Source: CAD feature listing. Evaluate the final solid. Frame: model axes, mm. Face numbers are marked on the shaded views. Coordinates: 2 decimals unless noted, no trailing zeros. Write each loop counter-clockwise with the first axis right and the second up, starting at its lowest first coordinate (ties: lowest second). Pieces come first, ordered by that corner, then holes. Notation, with made-up numbers: (68.25, 26.5) - (94.25, 26.5) arc R33 cw to (94.25, 56.5) - close; hole circle Ø1 at (51.5, 77). An arc over 180 degrees is marked (long way). One line per item, written item: value.
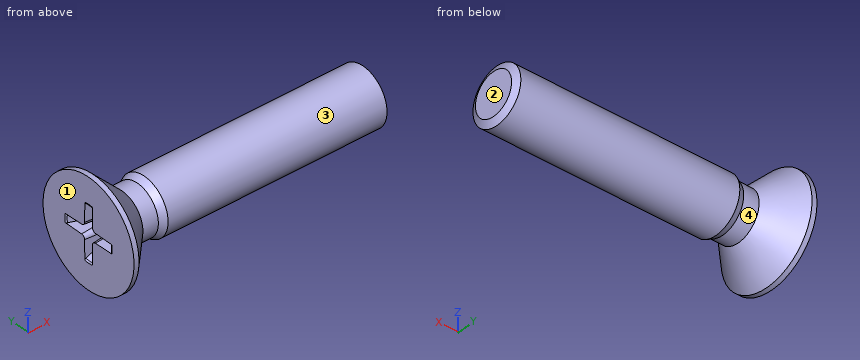
Autodesk Inventor part; units mm, degrees
ref_plane "Work Plane2" through (3.35, 0, 0) normal (0, 0, -1) x (1, 0, 0)
ref_plane "YZ Plane" through (0, 0, 0) normal (1, 0, 0) x (0, 1, 0)
ref_plane "XZ Plane" through (0, 0, 0) normal (0, 1, 0) x (-1, 0, 0)
sketch "Skizze1" plane through (0, 0, 0) normal (0, 0, 1) x (1, 0, 0)
  line L0 (1.2, 0) -> (10, 0)
  line L1 (10, 0) -> (10, 1)
  line L2 (10, 1) -> (2, 1)
  line L3 (2, 1) -> (1.7546, 0.8773)
  line L4 (1.7546, 0.8773) -> (1.2, 0.8773)
  line L5 (0, 1.9) -> (0, 0.95)
  line L6 (0, 0.95) -> (0.9455, 0.4786)
  line L7 (0.9455, 0.4786) -> (1.2, 0)
  line L8 (-2, 0) -> (12, 0)
  line L9 (0, -0.38) -> (0, 2.28)
  line L10 (0, 1.9) -> (0.1773, 1.9)
  line L11 (0.1773, 1.9) -> (1.2, 0.8773)
  line L12 (2, 1) -> (1.0773, 1) construction
  dimension "d1" = 8
  dimension "d2" = 2
  dimension "d3" = 1.7546
  dimension "d4" = 1.9
  dimension "d5" = 26.5
  dimension "d6" = 62
  dimension "d7" = 1.2
  dimension "d8" = 0.2454
  dimension "d12" = 3.8
  dimension "d13" = 45
  dimension "d15" = 10
  dimension "d24" = 1.2
revolve "Körper" add sketch "Skizze1" angle 360 about axis through (1.2, 0, 0) along (1, 0, 0) contours L7 L6 L5 L10 L11 L4 L3 L2 L1 L0
sketch "Skizze2" plane through (0, 0, 0) normal (-1, 0, 0) x (0, 0, 1)
  line L0 (0, 0.95) -> (0, 0) construction
  line L1 (0, 0) -> (0.95, 0) construction
  arc A0 (0.285, 0) -> (0, 0.285) centre (0, 0) ccw construction
  arc A1 (0.3325, 0) -> (0, 0.3325) centre (0, 0) ccw construction
  arc A2 (0.9373, 0.155) -> (0.155, 0.9373) centre (0, 0) ccw
  line L2 (0, 0) -> (0.6718, 0.6718) construction
  line L3 (0.155, 0.9373) -> (0.1646, 0.2889)
  line L4 (0.9373, 0.155) -> (0.2889, 0.1646)
  arc A3 (0.155, 0.9373) -> (0, 0.95) centre (0, 0) ccw
  arc A4 (0.95, 0) -> (0.9373, 0.155) centre (0, 0) ccw
  line L5 (0, -2.66) -> (0, 2.66)
  line L6 (-2.66, 0) -> (2.66, 0)
  arc A5 (0.155, -0.9373) -> (0.9373, -0.155) centre (0, 0) ccw
  line L7 (0.155, -0.9373) -> (0.1646, -0.2889)
  line L8 (0.9373, -0.155) -> (0.2889, -0.1646)
  arc A6 (0, -0.95) -> (0.155, -0.9373) centre (0, 0) ccw
  arc A7 (0.9373, -0.155) -> (0.95, 0) centre (0, 0) ccw
  arc A8 (-0.155, 0.9373) -> (-0.9373, 0.155) centre (0, 0) ccw
  line L9 (-0.155, 0.9373) -> (-0.1646, 0.2889)
  line L10 (-0.9373, 0.155) -> (-0.2889, 0.1646)
  arc A9 (0, 0.95) -> (-0.155, 0.9373) centre (0, 0) ccw
  arc A10 (-0.9373, 0.155) -> (-0.95, 0) centre (0, 0) ccw
  arc A11 (-0.155, -0.9373) -> (0, -0.95) centre (0, 0) ccw
  arc A12 (-0.9373, -0.155) -> (-0.155, -0.9373) centre (0, 0) ccw
  arc A13 (-0.95, 0) -> (-0.9373, -0.155) centre (0, 0) ccw
  line L11 (-0.9373, -0.155) -> (-0.2889, -0.1646)
  line L12 (-0.155, -0.9373) -> (-0.1646, -0.2889)
  arc A14 (0.1646, 0.2889) -> (0.2889, 0.1646) centre (0.2908, 0.2908) ccw
  arc A15 (0.2889, -0.1646) -> (0.1646, -0.2889) centre (0.2908, -0.2908) ccw
  arc A16 (-0.2889, 0.1646) -> (-0.1646, 0.2889) centre (-0.2908, 0.2908) ccw
  arc A17 (-0.1646, -0.2889) -> (-0.2889, -0.1646) centre (-0.2908, -0.2908) ccw
  point P0 (0.6718, -0.6718)
  point P1 (-0.6718, 0.6718)
  point P2 (-0.6718, -0.6718)
  dimension "d17" = 0.57
  dimension "d18" = 0.665
  dimension "d19" = 1.9
  dimension "d20" = 45
  dimension "d21" = 0.155
extrude "Loch" add sketch "Skizze2" against normal up to next draft 5 contours L4 A14 L3 A2 | A5 L7 A15 L8 | L9 A16 L10 A8 | A12 L11 A17 L12
fillet "Rundung1" radius 0.062 4 edges at (0, 0.95, 0) (0, 0, -0.95) (0, -0.95, 0) (0, 0, 0.95)
thread "Gewinde"
chamfer "Fase1" distance 0.2454 distance2 0.1227 1 edges at (10, -1, 0) measured on face at (10, -0.0858, 0.7069)
ref_plane "Work Plane2" through (3.35, 0, 0) normal (0, 0, -1) x (1, 0, 0)
equation "\"d1\" = GEL"
equation "\"d2\" = GD"
equation "\"d3\" = BDM"
equation "\"d4\" = SDM"
equation "\"d7\" = INTI"
equation "\"d8\" = GAL"
equation "\"d12\" = KOD"
equation "\"d13\" = 0.5 * SEWI"
equation "\"d15\" = NLG"
equation "\"d24\" = KOH"
equation "\"d17\" = 0.3 * SDM"
equation "\"d18\" = 0.35 * SDM"
equation "\"d19\" = SDM"
equation "\"d21\" = 0.5 * SBR"
equation "\"d23\" = 0.2 * SBR"
equation "\"d10\" = GEL"
equation "\"d25\" = -0.5 * SPD + 0.5 * GD"
equation "\"d26\" = 0.5 * GAL"
equation "\"NLG\" = 10"
equation "\"GEL\" = 8"
equation "\"GAL\" = 0.61345 * PTC"
equation "\"SPD\" = NND - 1.2269 * PTC"
equation "\"KOD\" = 3.8"
equation "\"KOH\" = 1.2"
equation "\"SBR\" = 0.31"
equation "\"INTI\" = 1.2"
equation "\"SDM\" = 1.9"
equation "\"GD\" = NND"
equation "\"BDM\" = NND - GAL"
equation "\"SEWI\" = 90deg"
equation "\"d9\" = SDM"
equation "\"GUL\" = 0.61345 * PTC"
equation "\"TOA\" = 30deg"
equation "\"EPV\" = 2.2"
equation "\"THREADDIA\" = 2"
equation "\"PTC\" = 0.4"
equation "\"NND\" = 2"
equation "\"GD1\" = THREADDIA - 1.2269 * PTC"
properties part number "ISO 7046-1 - M2 x 10 - 4.8 - H" material "Stahl"
1) Section query A-A on x = 8.25. Output: boundary loops of the cut face in (y, z), then the cut area to 3 significant figures.
Values found:
outline: circle Ø2 at (0, 0)
area: 3.14 mm2
2) Contact query for a flat-ended pin moving along its axis: P1, Ø2, axis at x = 7.5, y = -1, coming from the -Z side. Output: stop coordinate, or through.
Values found:
P1: z = -1
3) Material intervals for line 1 (Z direction, x = 7.75, y = 0); line 2 (Y direction, x = 8.75, z = 0.7); line 3 (X direction, y = -1.1, z = 0.4), sorted ascending.
Values found:
line 1: -1 to 1
line 2: -0.71 to 0.71
line 3: 0 to 0.91
4) Draft query along X for the marked faces 1, 2, 3 and 4. Return one class per face: released by +X, released by -X, zero draft, split by the parting line, or undercut.
Values found:
face 1: released by -X
face 2: released by +X
face 3: zero draft
face 4: undercut
